Build history of the part. All positions in model axes, mm. A direction names the side the tool comes from. Give positions to 0.01 mm unless a question says otherwise; leave off trailing zeros. Order: outer loops, then holes, each group sorted by start corner. A loop starts at its lowest first (then second) coordinate and runs counter-clockwise, first axis right, second up. Notation, with made-up numbers: (87, 30.5) - (122, 30.5) arc R15 ccw to (122, 39.5) - close; hole circle Ø5 at (68.5, 73). An arc over 180 degrees is marked (long way). Use a Markdown table: item, result.
from build123d import *

# Parameters (mm, degrees)
F0_W     = 174.4176968932
F0_H     = 211.885496974
F1_DEPTH = 80.772
F2_T     = -2.54
F3_W     = 186.191752553
F3_H     = 5.066819489
F4_DEPTH = 11.938


with BuildPart() as f1:
    # F0 (on Top) → F1 (new body)
    with BuildSketch(Plane.XY):
        with Locations((-0.6318576634, 1.6548894346)):
            Rectangle(F0_W, F0_H)
    extrude(amount=F1_DEPTH)

    # F2
    f2_openings = [f1.faces().sort_by_distance(p)[0] for p in [
        (-0.631858, 1.654889, 80.772),
    ]]
    offset(amount=F2_T, openings=f2_openings)

    # F3 (on face) → F4 (cut)
    with BuildSketch(Plane(origin=(-87.84070611, 0, 0), x_dir=(0, -1, 0), z_dir=(-1, 0, 0))):
        with Locations((-1.3709291816, 70.3899897635)):
            Rectangle(F3_W, F3_H)
    extrude(amount=-F4_DEPTH, mode=Mode.SUBTRACT)


solid = f1.part
1) Slice it at C-C (x = -68). Write the cut outline in (y, z), and give its area (3 significant figures).
Computed:
| item | result |
|---|---|
| outline | (-104.29, 0) - (107.6, 0) - (107.6, 80.77) - (105.06, 80.77) - (105.06, 2.54) - (-101.75, 2.54) - (-101.75, 80.77) - (-104.29, 80.77) - close |
| area | 936 mm² |
2) Two-plate mould, pull along X, no slides. Class faces 3 (the flat face through (-2, 3, 0)), 4 (the flat face through (-2, 105.058, 41)), 5 (the flat face through (-87.841, 0, 40)): +X half, -X half, draft (parallel to the pull), parting line (faces both ways), or undercut.
Computed:
| item | result |
|---|---|
| face 3 | draft |
| face 4 | undercut |
| face 5 | -X half |
3) Pin check, flat tip, straight feed: P1, Ø8, axis at x = 23.5, y = 46, coming from the +Z side. Stop position of the tip, or through.
Computed:
| item | result |
|---|---|
| P1 | stops at z = 2.54 |
4) Tool access for faces 1 (the flat face through (-2, 3, 2.54)), 2 (the flat face through (-2, 107.598, 40)): list every direction of +Z, -Z, +X, -X, +Y, -Y with a clear straight run to the whole face (end or side of a thin tool).
Computed:
| item | result |
|---|---|
| face 1 | +Z |
| face 2 | +Z, -Z, +X, -X, +Y |
5) Slice it at A-A (y = -27). Write the cut outline in (x, z).
Computed:
| item | result |
|---|---|
| outline | (-87.84, 0) - (86.58, 0) - (86.58, 80.77) - (84.04, 80.77) - (84.04, 2.54) - (-85.3, 2.54) - (-85.3, 67.86) - (-87.84, 67.86) - close; (-87.84, 72.92) - (-85.3, 72.92) - (-85.3, 80.77) - (-87.84, 80.77) - close |
6) Slice it at B-B (z = 48.5). Write the cut outline in (x, y), and give its area (3 significant figures).
Computed:
| item | result |
|---|---|
| outline | (-87.84, -104.29) - (86.58, -104.29) - (86.58, 107.6) - (-87.84, 107.6) - close; hole (-85.3, -101.75) - (84.04, -101.75) - (84.04, 105.06) - (-85.3, 105.06) - close |
| area | 1,940 mm² |
7) Wall check: line 1 (X direction, y = -58, z = 63.5); line 2 (Y direction, x = -19, z = 33); line 3 (Z direction, x = -68, y = -70.5). Give the ranges that are in metal, low to high. Write a range as from..to.
Computed:
| item | result |
|---|---|
| line 1 | x = -87.84..-85.3, 84.04..86.58 |
| line 2 | y = -104.29..-101.75, 105.06..107.6 |
| line 3 | z = 0..2.54 |
